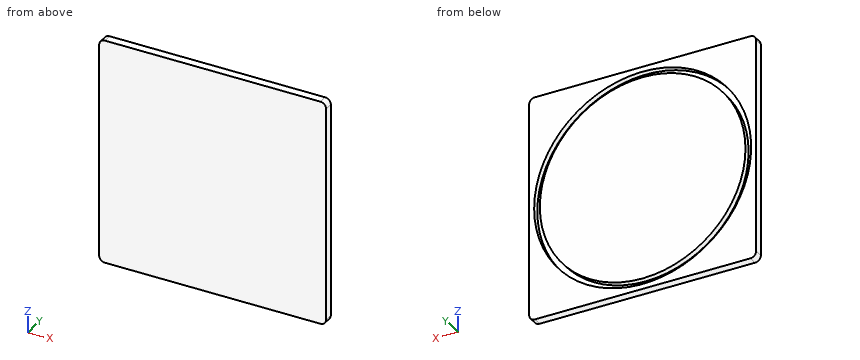
```python
from build123d import *

# Parameters (mm, degrees)
SKETCH1_W               = 80
SKETCH1_H               = 80
BOSS_EXTRUDE1_DEPTH     = 3
SKETCH3_R               = 38.25
SKETCH3_R_2             = 36.25
CUT_EXTRUDE_THIN1_DEPTH = 2
FILLET1_R               = 2


with BuildPart() as part:
    # Sketch1 → Boss-Extrude1 (new body)
    with BuildSketch(Plane(origin=(0, 0, 0), x_dir=(1, 0, 0), z_dir=(0, 1, 0))):
        with Locations((40, 0)):
            Rectangle(SKETCH1_W, SKETCH1_H)
    extrude(amount=BOSS_EXTRUDE1_DEPTH)

    # Sketch3 → Cut-Extrude-Thin1 (cut)
    with BuildSketch(Plane(origin=(0, 3, 0), x_dir=(1, 0, 0), z_dir=(0, 1, 0))):
        with Locations((40, 0)):
            Circle(SKETCH3_R)
        with Locations((40, 0)):
            Circle(SKETCH3_R_2, mode=Mode.SUBTRACT)
    extrude(amount=-CUT_EXTRUDE_THIN1_DEPTH, mode=Mode.SUBTRACT)

    # Fillet1
    fillet1_edges = [part.edges().sort_by_distance(p)[0] for p in [
        (80, 1.5, -40),
        (80, 1.5, 40),
        (0, 1.5, 40),
        (0, 1.5, -40),
    ]]
    fillet(fillet1_edges, radius=FILLET1_R)


solid = part.part
```
Model file for the job. Use its own axes, mm. Coordinates: 2 decimals unless noted, no trailing zeros. Loops run counter-clockwise (first coordinate to the right, second up) from the corner with the lowest first, then second, coordinate; pieces in that order, holes last. Notation, with made-up numbers: (-22, -29) - (36, -29) arc R20 ccw to (36, -6) - close; hole circle Ø10 at (17.25, 66.25). An arc over 180 degrees is marked (long way). Answer as a JSON object with one key per item and string values. Group by question number.
(1) Cut at A-A (y = 2.5). Give the cut face in (x, z).
(2) Cut at B-B (x = 40). Give the cut face in (y, z).
(3) Probe line 1 along X through (y, z) = (1.65, 0); line 2 along Z through (x, y) = (40, 2.5); line 3 along X through (y, z) = (1.1, -4). List the from-to ranges inside material, lowest first.
(4) Cut at C-C (z = 0). Give the cut face in (x, y), then the cut area to 3 significant figures.
Geometry says:
{
 "1": {"outline": "(0, -38) arc R2 ccw to (2, -40) - (78, -40) arc R2 ccw to (80, -38) - (80, 38) arc R2 ccw to (78, 40) - (2, 40) arc R2 ccw to (0, 38) - close; circle Ø72.5 at (40, 0); hole circle Ø76.5 at (40, 0)"},
 "2": {"outline": "(0, -40) - (3, -40) - (3, -38.25) - (1, -38.25) - (1, -36.25) - (3, -36.25) - (3, 36.25) - (1, 36.25) - (1, 38.25) - (3, 38.25) - (3, 40) - (0, 40) - close"},
 "3": {"line 1": "x = 0 to 1.75, 3.75 to 76.25, 78.25 to 80", "line 2": "z = -40 to -38.25, -36.25 to 36.25, 38.25 to 40", "line 3": "x = 0 to 1.96, 3.97 to 76.03, 78.04 to 80"},
 "4": {"outline": "(0, 0) - (80, 0) - (80, 3) - (78.25, 3) - (78.25, 1) - (76.25, 1) - (76.25, 3) - (3.75, 3) - (3.75, 1) - (1.75, 1) - (1.75, 3) - (0, 3) - close", "area": "232 mm^2"}
}
